Model file for the job. Use its own axes, mm. Face numbers are marked on the shaded views. A direction names the side the tool comes from. Coordinates: 2 decimals unless noted, no trailing zeros. Write each loop counter-clockwise with the first axis right and the second up, starting at its lowest first coordinate (ties: lowest second). Pieces come first, ordered by that corner, then holes. Notation, with made-up numbers: (64, 25.25) - (82, 25.25) arc R17 cw to (82, 48.25) - close; hole circle Ø5 at (7.5, 59.25). An arc over 180 degrees is marked (long way). Put each result on its own line as item: value. Start each with the question number.
1. Pull direction Y, two halves, no side cores. Call the marked faces 4, 5 and 6: released by +Y, released by -Y, zero draft, split by the parting line, or undercut.
2. Saw through at B-B, the plane z = 0. Write the cut outline in (x, y) (3 decimals), plus the area to 3 significant figures.
3. Drill centre lines: L1, parallel to Y at x = 0, z = 3; L2, parallel to Y at x = -15.5, z = -13.5; L3, parallel to Z at x = -8, y = 15. Where is each one in solid material? Low to high. Write a range as from..to.
4. Drop flat-ended pins along their axis: P1, Ø1.8, axis at x = 2, z = 0.5, coming from the -Y side (3 decimals); P2, Ø0.5, axis at x = -24.5, y = 31.5, coming from the -Z side; P3, Ø2, axis at x = -13, z = 9.5, coming from the -Y side. Give the stop position or say it passes through.
5. Which spindle directions (+Z, -Z, +X, -X, +Y, -Y) get a long thin tool onto all of the face, cutting with end or side? Do the marked faces 1, 2 and 3. Say none if no direction does.
6. Saw through at A-A, the plane x = 0. Give the number of separate pieces and of enclosed holes in the cut face, plus the area to 3 significant figures.
7. Saw through at C-C, the plane y = 23. Write the cut outline in (x, z).
8. Saw through at D-D, the plane x = 12.7. Write the cut outline in (y, z), plus the area to 3 significant figures.
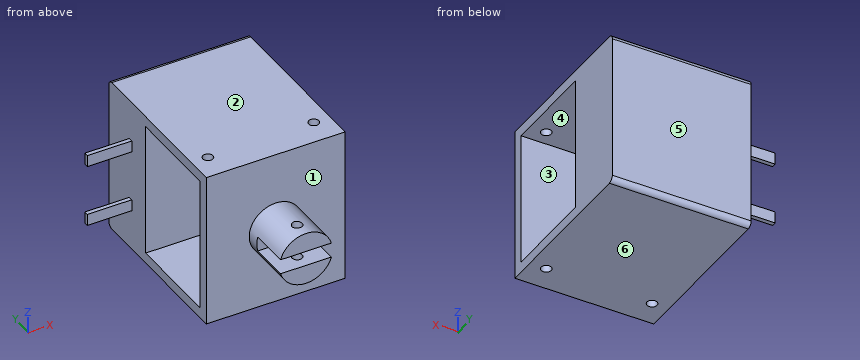
Autodesk Fusion 360 part; units mm, degrees
sketch "Sketch1" plane through (0, 0, 0) normal (0, 1, 0) x (1, 0, 0)
  line L0 (16.6624, -18.6436) -> (-16.6624, -18.6436)
  line L1 (-16.6624, -18.6436) -> (-16.6624, 18.6436)
  line L2 (-16.6624, 18.6436) -> (16.6624, 18.6436)
  line L3 (16.6624, 18.6436) -> (16.6624, -18.6436)
  line L4 (16.6624, -18.6436) -> (-16.6624, 18.6436) construction
  line L5 (-16.6624, -18.6436) -> (16.6624, 18.6436) construction
  dimension "d1" = 33.3248
  dimension "d2" = 37.2872
extrude "Extrude1" add sketch "Sketch1" along normal blind 40.8686
cylinder "CylinderPrimitive1" add diameter 12.7 height -12.7 placed x (1, 0, 0) y (0, 0, -1) z (0, 1, 0) at (0, 0, 0)
sketch "Sketch3" plane through (0, -12.7, 0) normal (0, -1, 0) x (1, 0, 0)
  circle A0 centre (0, 0) radius 6.35
  line L0 (-6.35, -1.778) -> (6.35, -1.778)
  arc A1 (6.35, -1.778) -> (6.35, 1.778) centre (6.35, 0) ccw
  line L1 (6.35, 1.778) -> (-6.35, 1.778)
  arc A2 (-6.35, 1.778) -> (-6.35, -1.778) centre (-6.35, 0) ccw
  line L2 (-6.35, 0) -> (6.35, 0) construction
extrude "Extrude2" cut sketch "Sketch3" against normal blind 9.525 contours A0 L0 L1
fillet "Fillet1" radius 1.27 2 edges at (0, 40.8686, 18.6436) (0, 40.8686, -18.6436)
hole "Hole1" at (0, -9.0033, -6.35) direction (0, 0, 1) diameter 2.4384 depth 37.2872 tip angle 180
sketch "Sketch4" plane through (0, 0, -18.6436) normal (0, 0, -1) x (-1, 0, 0)
  line L0 (16.6624, 39.5986) -> (-16.6624, 39.5986)
  line L1 (-16.6624, 39.5986) -> (-16.6624, 0)
  line L2 (-16.6624, 0) -> (16.6624, 0)
  line L3 (16.6624, 0) -> (16.6624, 39.5986)
  line L4 (0, 0) -> (0, 6.223)
  line L5 (0, 6.223) -> (12.7, 6.223)
  line L6 (12.7, 6.223) -> (0, 6.223)
  line L7 (0, 6.223) -> (-12.7, 6.223)
  dimension "d13" = 6.223
  dimension "d14" = 12.7
hole "Hole2" at (12.7, 6.223, -18.6436) direction (0, 0, 1) diameter 2.4384 depth 37.2872 tip angle 180
mirror "Mirror1" about plane through (0, 0, 0) normal (1, 0, 0) of "Hole2"
sketch "Sketch5" plane through (-16.6624, 0, 0) normal (-1, 0, 0) x (0, 0, 1)
  arc A0 (-17.3736, 40.8686) -> (-18.6436, 39.5986) centre (-17.3736, 39.5986) ccw
  line L0 (-18.6436, 39.5986) -> (-18.6436, 0)
  line L1 (-18.6436, 0) -> (18.6436, 0)
  line L2 (18.6436, 0) -> (18.6436, 39.5986)
  arc A1 (18.6436, 39.5986) -> (17.3736, 40.8686) centre (17.3736, 39.5986) ccw
  line L3 (17.3736, 40.8686) -> (-17.3736, 40.8686)
  line L4 (-16.1036, 25.4052) -> (16.1036, 25.4052)
  line L5 (16.1036, 25.4052) -> (16.1036, 2.54)
  line L6 (16.1036, 2.54) -> (-16.1036, 2.54)
  line L7 (-16.1036, 2.54) -> (-16.1036, 25.4052)
  line L8 (16.1036, 13.9726) -> (18.6436, 13.9726) construction
  line L9 (-16.1036, 13.9726) -> (-18.6436, 13.9802) construction
  line L10 (0, 2.54) -> (0, 0) construction
  line L11 (0, 25.4052) -> (0, 40.8686) construction
extrude "Extrude3" cut sketch "Sketch5" against normal blind 30.8102 contours L4 L5 L6 L7
sketch "Sketch6" plane through (-16.6624, 0, 0) normal (-1, 0, 0) x (0, 0, 1)
  line L0 (16.1036, 25.4052) -> (16.1036, 2.54)
  line L1 (16.1036, 2.54) -> (-16.1036, 2.54)
  line L2 (-16.1036, 2.54) -> (-16.1036, 25.4052)
  line L3 (-16.1036, 25.4052) -> (16.1036, 25.4052)
  arc A0 (-17.3736, 40.8686) -> (-18.6436, 39.5986) centre (-17.3736, 39.5986) ccw
  line L4 (-18.6436, 39.5986) -> (-18.6436, 0)
  line L5 (-18.6436, 0) -> (18.6436, 0)
  line L6 (18.6436, 0) -> (18.6436, 39.5986)
  arc A1 (18.6436, 39.5986) -> (17.3736, 40.8686) centre (17.3736, 39.5986) ccw
  line L7 (17.3736, 40.8686) -> (-17.3736, 40.8686)
  line L8 (0, 40.8686) -> (0, 31.75) construction
  line L9 (0, 31.75) -> (7.493, 31.75) construction
  line L10 (8.89, 32.258) -> (6.096, 32.258)
  line L11 (6.096, 32.258) -> (6.096, 31.242)
  line L12 (6.096, 31.242) -> (8.89, 31.242)
  line L13 (8.89, 31.242) -> (8.89, 32.258)
  line L14 (8.89, 32.258) -> (6.096, 31.242) construction
  line L15 (6.096, 32.258) -> (8.89, 31.242) construction
  dimension "d21" = 7.493
extrude "Extrude4" add sketch "Sketch6" along normal blind 10.668 contours L10 L11 L12 L13
mirror "Mirror2" about plane through (0, 0, 0) normal (0, 0, 1) of "Extrude4"
extrude "Extrude5" cut 1 faces at (14.1478, 17.7834, 5.3679) along direction (1, 0, 0) blind 7.62
Final values:
1. face 4: undercut
1. face 5: released by +Y
1. face 6: zero draft
2. outline: (-16.662, 0) - (-6.35, 0) - (-6.35, -3.175) - (6.35, -3.175) - (6.35, 0) - (16.662, 0) - (16.662, 2.54) - (-16.662, 2.54) - close; (-16.662, 25.405) - (16.662, 25.405) - (16.662, 40.869) - (-16.662, 40.869) - close
2. area: 640 mm²
3. L1: y = -12.7..-10.22, -7.78..2.54, 25.41..40.87
3. L2: y = 0..2.54, 25.41..40.87
3. L3: z = -18.64..-16.1, 16.1..18.64
4. P1: stops at y = -3.175
4. P2: stops at z = -8.89
4. P3: stops at y = 0
5. face 1: -Y
5. face 2: +Z, +X, -X, +Y, -Y
5. face 3: +X, -X
6. separate pieces: 3
6. enclosed holes: 1
6. area: 892 mm²
7. outline: (-16.66, -18.64) - (16.66, -18.64) - (16.66, -16.1) - (-16.66, -16.1) - close; (-16.66, 16.1) - (16.66, 16.1) - (16.66, 18.64) - (-16.66, 18.64) - close
8. outline: (0, -18.64) - (5, -18.64) - (5, -16.1) - (2.54, -16.1) - (2.54, 16.1) - (5, 16.1) - (5, 18.64) - (0, 18.64) - close; (7.44, -18.64) - (39.6, -18.64) arc R1.27 ccw to (40.87, -17.37) - (40.87, 17.37) arc R1.27 ccw to (39.6, 18.64) - (7.44, 18.64) - (7.44, 16.1) - (25.41, 16.1) - (25.41, -16.1) - (7.44, -16.1) - close
8. area: 774 mm²
